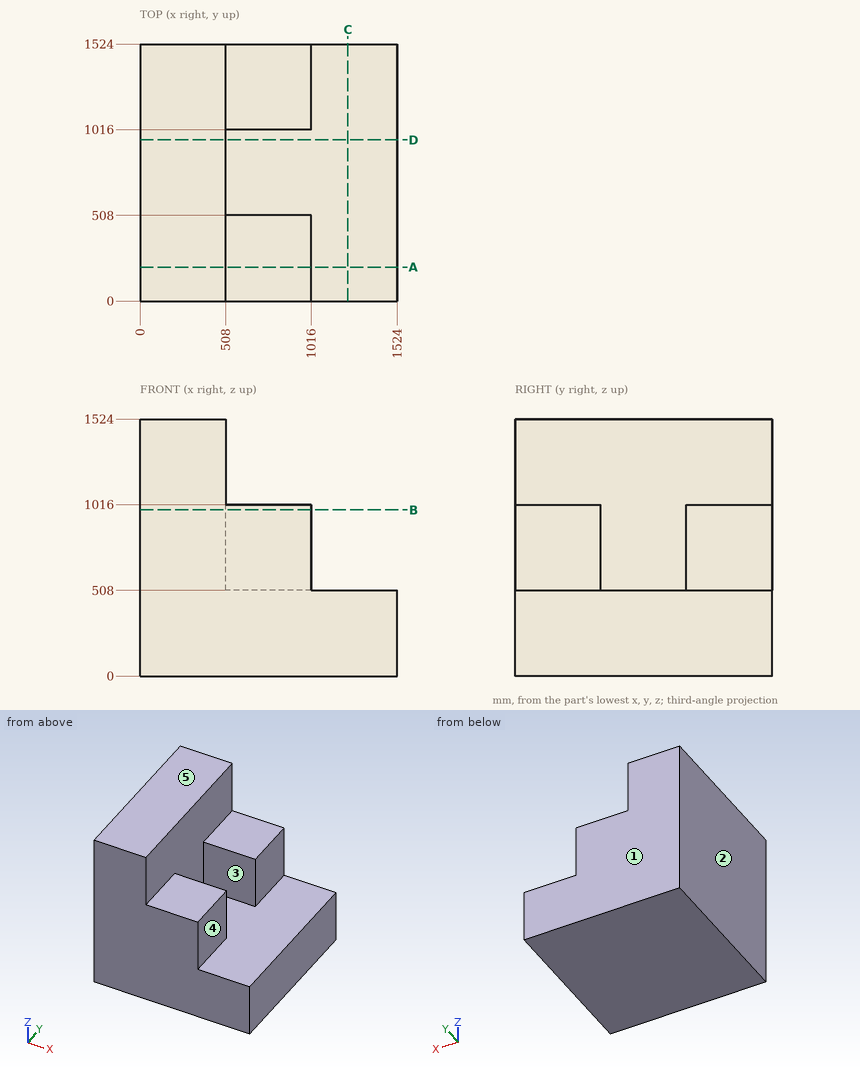
Study the drawing (mm; zero at the part's minimum x, y, z) and answer. A direction names the side the tool comes from. Round coordinates to 2 decimals unless told otherwise and drop trailing zeros. Loops run counter-clockwise (first coordinate to the right, second up) from the corner with the lowest first, then second, coordinate; pieces in that order, holes last. Notation, with made-up numbers: (44, -30.75) -> (77, -30.75) arc R30 cw to (77, 0.25) -> close; hole circle Ø1 at (45.5, 73.25). An arc over 180 degrees is marked (long way). Write each question's results on one line, items separated by ' | '. Start each with the question number.
1. Given pin 1 Ø3 at (x, y) = (1199.5, 1159) entering from +Z; pin 2 Ø5 at (x, z) = (262, 821.5) entering from -Y; pin 3 Ø6 at (y, z) = (939.5, 763.5) entering from +X, each flat-ended and moving along its own axis, determine where each tip first touches the part or whether it passes through.
2. Section A-A (y = 200.5) is taken. Determine the outline of the cut face in (x, z), plus the area to 3 significant figures.
3. Section C-C (x = 1232) is taken. Determine the outline of the cut face in (y, z), plus the area to 3 significant figures.
4. Find the intervals of material crossed by probe 1 along Z at (x, y) = (788.5, 541); probe 2 along Z at (x, y) = (626.5, 467), in increasing order. Write a range as from..to.
5. A tool of negligible diameter and unlimited length cuts with its end or side. For the marked faces 4 and 5, from which of +Z, -Z, +X, -X, +Y, -Y can it reach the whole face along a straight path? Write none if from no direction.
6. For a pull along Y with two mould halves and no side action, classify the marked faces 1, 2 and 3 as +Y half, -Y half, draft (parallel to the pull), parting line (faces both ways), or undercut.
7. Section B-B (z = 985.5) is taken. Determine the outline of the cut face in (x, y), plus the area to 3 significant figures.
8. Section D-D (y = 955.5) is taken. Determine the outline of the cut face in (x, z), plus the area to 3 significant figures.
Evaluation:
1) pin 1: stops at z = 508 | pin 2: stops at y = 0 | pin 3: stops at x = 508
2) outline: (0, 0) -> (1524, 0) -> (1524, 508) -> (1016, 508) -> (1016, 1016) -> (508, 1016) -> (508, 1524) -> (0, 1524) -> close | area: 1,550,000 mm2
3) outline: (0, 0) -> (1524, 0) -> (1524, 508) -> (0, 508) -> close | area: 774,000 mm2
4) probe 1: z = 0..508 | probe 2: z = 0..1016
5) face 4: +Z, +X, +Y, -Y | face 5: +Z, +X, -X, +Y, -Y
6) face 1: +Y half | face 2: draft | face 3: undercut
7) outline: (0, 0) -> (1016, 0) -> (1016, 508) -> (508, 508) -> (508, 1016) -> (1016, 1016) -> (1016, 1524) -> (0, 1524) -> close | area: 1,290,000 mm2
8) outline: (0, 0) -> (1524, 0) -> (1524, 508) -> (508, 508) -> (508, 1524) -> (0, 1524) -> close | area: 1,290,000 mm2
